Part model, mm, in its own coordinate system. Face numbers are marked on the shaded views. A direction names the side the tool comes from. Round coordinates to 2 decimals unless told otherwise and drop trailing zeros. Write each loop counter-clockwise with the first axis right and the second up, starting at its lowest first coordinate (ties: lowest second). Pieces come first, ordered by that corner, then holes.
1) Saw through at B-B on y = 17. Write the cut outline in (x, z), and give its area (3 significant figures).
2) Drill centre lines: L1, parallel to Y at x = 34.1, z = 8; L2, parallel to Z at x = 34.2, y = 17; L3, parallel to Y at x = 10.5, z = -1.6. Where is each one in solid material? Low to high.
3) Flat gauge pins, fed straight in: pin 1 (1 mm diameter, centred on x = 18, y = 10.5, fed in from +Z); pin 2 (10 mm diameter, centred on x = 24, y = 19.5, fed in from +Z); pin 3 (3.5 mm diameter, centred on y = 16, z = 6, fed in from -X); pin 4 (4.5 mm diameter, centred on y = 17, z = 8, fed in from +X). Where does each tip first touch, or does it go through?
4) Saw through at C-C on x = 3.5. Write the cut outline in (y, z), and give its area (3 significant figures).
5) Saw through at A-A on z = 8. Write the cut outline in (x, y).
6) Which spindle directions (+Z, -Z, +X, -X, +Y, -Y) get a long thin tool onto all of the face, cutting with end or side? Do the marked faces 4 and 5. Say none if no direction does.
7) Pull direction Z, two halves, no side cores. Call the marked faces 1, 2 and 3: +Z half, -Z half, draft (parallel to the pull), parting line (faces both ways), or undercut.
8) Saw through at D-D on y = 10. Write the cut outline in (x, z), and give its area (3 significant figures).
```python
from build123d import *

# Parameters (mm, degrees)
SKIZZE1_W                                            = 34
SKIZZE1_H                                            = 14
BASIS_BLECH1_DEPTH                                   = 2
KANTE_LASCHE1_STRIP_W                                = 12
KANTE_LASCHE1_STRIP_H                                = 2
KANTE_LASCHE1_STRIP_CUT_DEPTH                        = 14
KANTE_LASCHE1_DEPTH                                  = 14
KANTE_LASCHE1_START                                  = 2
KANTE_LASCHE1_FLAT_DEPTH                             = 2
SKIZZE10_R                                           = 1.7
SCHNITT_LINEAR_AUSTRAGEN1_DEPTH                      = 45.147480109
FORMSENKUNG_F_R_M3_SENKSCHRAUBE_MIT_INNE_D           = 3.4
FORMSENKUNG_F_R_M3_SENKSCHRAUBE_MIT_INNE_CSINK_D     = 6.94
FORMSENKUNG_F_R_M3_SENKSCHRAUBE_MIT_INNE_CSINK_ANGLE = 90


# Sheet-metal steps are written as plain solids
with BuildPart() as part:
    # Skizze1 → Basis-Blech1 (new body)
    with BuildSketch(Plane.XY):
        with Locations((17, 7)):
            Rectangle(SKIZZE1_W, SKIZZE1_H)
    extrude(amount=-BASIS_BLECH1_DEPTH)

    # Kante-Lasche1 strip (across the edge) → Kante-Lasche1 strip cut (cut)
    with BuildSketch(Plane(origin=(34, 0, 0), x_dir=(-1, 0, 0), z_dir=(0, 1, 0))):
        with Locations((-4, -1)):
            Rectangle(KANTE_LASCHE1_STRIP_W, KANTE_LASCHE1_STRIP_H)
    extrude(amount=KANTE_LASCHE1_STRIP_CUT_DEPTH, mode=Mode.SUBTRACT)

    # Kante-Lasche1 bend section (across the edge) → Kante-Lasche1 (add)
    with BuildSketch(Plane(origin=(34, 0, 0), x_dir=(-1, 0, 0), z_dir=(0, 1, 0))):
        with BuildLine():
            Line((-2, 2), (0, 2))
            ThreePointArc((0, 2), (0.585786438, 0.585786438), (2, 0))
            Line((2, 0), (2, -2))
            ThreePointArc((2, -2), (-0.828427125, -0.828427125), (-2, 2))
        make_face()
    extrude(amount=KANTE_LASCHE1_DEPTH)

    # Kante-Lasche1 profile (on flange) → Kante-Lasche1 flat (add)
    with BuildSketch(Plane.YZ.offset(34).offset(KANTE_LASCHE1_START)):
        Polygon((0, 13), (0, 2), (14, 2), (14, 3), (22, 3), (22, 13), align=None)
    extrude(amount=-KANTE_LASCHE1_FLAT_DEPTH)

    # Skizze10 → Schnitt-Linear austragen1 (cut, through all)
    with BuildSketch(Plane.XY):
        with Locations((3.5, 7)):
            Circle(SKIZZE10_R)
        with Locations((10.5, 7)):
            Circle(SKIZZE10_R)
    extrude(amount=-SCHNITT_LINEAR_AUSTRAGEN1_DEPTH, mode=Mode.SUBTRACT)

    # Formsenkung für M3 Senkschraube mit Innensechskant1 (through all)
    with Locations(Plane(origin=(36, 0, 0), x_dir=(0, 0, -1), z_dir=(1, 0, 0))):
        with Locations((-8, 5), (-8, 17)):
            CounterSinkHole(FORMSENKUNG_F_R_M3_SENKSCHRAUBE_MIT_INNE_D / 2, FORMSENKUNG_F_R_M3_SENKSCHRAUBE_MIT_INNE_CSINK_D / 2, counter_sink_angle=FORMSENKUNG_F_R_M3_SENKSCHRAUBE_MIT_INNE_CSINK_ANGLE)


solid = part.part
```
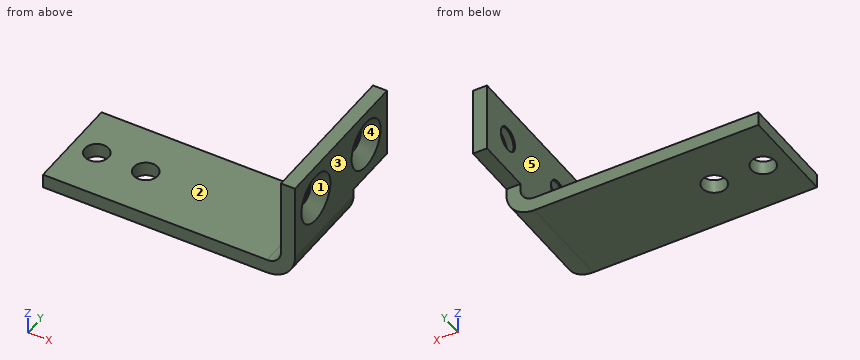
Completed:
1. outline: (34, 3) - (36, 3) - (36, 4.53) - (34.23, 6.3) - (34, 6.3) - close; (34, 9.7) - (34.23, 9.7) - (36, 11.47) - (36, 13) - (34, 13) - close
1. area: 10.1 mm2
2. L1: y = 0 to 3.3, 6.7 to 15.3, 18.7 to 22
2. L2: z = 3 to 6.3, 9.7 to 13
2. L3: y = 0 to 5.3, 8.7 to 14
3. pin 1: stops at z = 0
3. pin 2: passes through
3. pin 3: stops at x = 34
3. pin 4: stops at x = 34.78
4. outline: (0, -2) - (5.3, -2) - (5.3, 0) - (0, 0) - close; (8.7, -2) - (14, -2) - (14, 0) - (8.7, 0) - close
4. area: 21.2 mm2
5. outline: (34, 0) - (36, 0) - (36, 1.53) - (34.23, 3.3) - (34, 3.3) - close; (34, 6.7) - (34.23, 6.7) - (36, 8.47) - (36, 13.53) - (34.23, 15.3) - (34, 15.3) - close; (34, 18.7) - (34.23, 18.7) - (36, 20.47) - (36, 22) - (34, 22) - close
6. face 4: +X
6. face 5: +Z, -X, +Y, -Y
7. face 1: undercut
7. face 2: +Z half
7. face 3: draft
8. outline: (0, -2) - (32, -2) arc R4 ccw to (36, 2) - (36, 13) - (34, 13) - (34, 2) arc R2 cw to (32, 0) - (0, 0) - close
8. area: 95.4 mm2
